from build123d import *

# Parameters (mm, degrees)
SKETCH2_R           = 100
SKETCH2_R_2         = 4
BOSS_EXTRUDE1_DEPTH = 2
SKETCH3_R           = 65
SKETCH3_R_2         = 61
CUT_EXTRUDE2_DEPTH  = 1
CUT_EXTRUDE3_DEPTH  = 10


with BuildPart() as part:
    # Sketch2 → Boss-Extrude1 (new, symmetric)
    with BuildSketch(Plane(origin=(0, 0, 0), x_dir=(1, 0, 0), z_dir=(0, 1, 0))):
        with Locations(Location((0, 0, 0), (0, 0, 270))):
            Circle(SKETCH2_R)
        with Locations(Location((50, 0, 0), (0, 0, 270))):
            Circle(SKETCH2_R_2, mode=Mode.SUBTRACT)
        with Locations(Location((-25, -43.301270189, 0), (0, 0, 270))):
            Circle(SKETCH2_R_2, mode=Mode.SUBTRACT)
        with Locations(Location((-25, 43.301270189, 0), (0, 0, 270))):
            Circle(SKETCH2_R_2, mode=Mode.SUBTRACT)
        with BuildLine():
            ThreePointArc((-36.718407842, 33.937568056), (-17.5, 30.310889132), (-11.031592158, 48.767858006))
            ThreePointArc((-11.031592158, 48.767858006), (25, 43.301270189), (47.75, 14.83028995))
            ThreePointArc((47.75, 14.83028995), (35, 0), (47.75, -14.83028995))
            ThreePointArc((47.75, -14.83028995), (25, -43.301270189), (-11.031592158, -48.767858006))
            ThreePointArc((-11.031592158, -48.767858006), (-17.5, -30.310889132), (-36.718407842, -33.937568056))
            ThreePointArc((-36.718407842, -33.937568056), (-50, 0), (-36.718407842, 33.937568056))
        make_face(mode=Mode.SUBTRACT)
    extrude(amount=BOSS_EXTRUDE1_DEPTH, both=True)

    # Sketch3 → Cut-Extrude2 (cut)
    with BuildSketch(Plane(origin=(0, 2, 0), x_dir=(1, 0, 0), z_dir=(0, 1, 0))):
        with Locations(Location((0, 0, 0), (0, 0, 270))):
            Circle(SKETCH3_R)
        with Locations(Location((0, 0, 0), (0, 0, 270))):
            Circle(SKETCH3_R_2, mode=Mode.SUBTRACT)
    extrude(amount=-CUT_EXTRUDE2_DEPTH, mode=Mode.SUBTRACT)

    # Sketch4 → Cut-Extrude3 (cut)
    with BuildSketch(Plane(origin=(0, 2, 0), x_dir=(1, 0, 0), z_dir=(0, 1, 0))):
        with BuildLine():
            Line((6.221861376, 81.776580022), (7.721861376, 84.374656233))
            ThreePointArc((7.721861376, 84.374656233), (11.819937588, 85.472732444), (12.918013799, 81.374656233))
            Line((12.918013799, 81.374656233), (11.418013799, 78.776580022))
            ThreePointArc((11.418013799, 78.776580022), (7.319937588, 77.67850381), (6.221861376, 81.776580022))
        make_face()
        with BuildLine():
            Line((0.221861376, 71.384275176), (1.721861376, 73.982351387))
            ThreePointArc((1.721861376, 73.982351387), (5.819937588, 75.080427599), (6.918013799, 70.982351387))
            Line((6.918013799, 70.982351387), (5.418013799, 68.384275176))
            ThreePointArc((5.418013799, 68.384275176), (1.319937588, 67.286198965), (0.221861376, 71.384275176))
        make_face()
        with BuildLine():
            Line((18.918013799, 91.766961078), (17.418013799, 89.168884867))
            ThreePointArc((17.418013799, 89.168884867), (13.319937588, 88.070808656), (12.221861376, 92.168884867))
            Line((12.221861376, 92.168884867), (13.721861376, 94.766961078))
            ThreePointArc((13.721861376, 94.766961078), (17.819937588, 95.86503729), (18.918013799, 91.766961078))
        make_face()
        with BuildLine():
            Line((-53.425253905, 62.224294646), (-54.20171104, 65.122072125))
            ThreePointArc((-54.20171104, 65.122072125), (-52.080390696, 68.796306739), (-48.406156082, 66.674986396))
            Line((-48.406156082, 66.674986396), (-47.629698947, 63.777208917))
            ThreePointArc((-47.629698947, 63.777208917), (-49.75101929, 60.102974303), (-53.425253905, 62.224294646))
        make_face()
        with BuildLine():
            Line((-50.319425363, 50.633184731), (-51.095882499, 53.53096221))
            ThreePointArc((-51.095882499, 53.53096221), (-48.974562155, 57.205196824), (-45.300327541, 55.08387648))
            Line((-45.300327541, 55.08387648), (-44.523870406, 52.186099001))
            ThreePointArc((-44.523870406, 52.186099001), (-46.645190749, 48.511864387), (-50.319425363, 50.633184731))
        make_face()
        with BuildLine():
            Line((-51.511984623, 78.266096311), (-50.735527488, 75.368318832))
            ThreePointArc((-50.735527488, 75.368318832), (-52.856847832, 71.694084218), (-56.531082446, 73.815404562))
            Line((-56.531082446, 73.815404562), (-57.307539581, 76.713182041))
            ThreePointArc((-57.307539581, 76.713182041), (-55.186219238, 80.387416655), (-51.511984623, 78.266096311))
        make_face()
        with BuildLine():
            Line((-81.776580022, 6.221861376), (-84.374656233, 7.721861376))
            ThreePointArc((-84.374656233, 7.721861376), (-85.472732444, 11.819937588), (-81.374656233, 12.918013799))
            Line((-81.374656233, 12.918013799), (-78.776580022, 11.418013799))
            ThreePointArc((-78.776580022, 11.418013799), (-77.67850381, 7.319937588), (-81.776580022, 6.221861376))
        make_face()
        with BuildLine():
            Line((-71.384275176, 0.221861376), (-73.982351387, 1.721861376))
            ThreePointArc((-73.982351387, 1.721861376), (-75.080427599, 5.819937588), (-70.982351387, 6.918013799))
            Line((-70.982351387, 6.918013799), (-68.384275176, 5.418013799))
            ThreePointArc((-68.384275176, 5.418013799), (-67.286198965, 1.319937588), (-71.384275176, 0.221861376))
        make_face()
        with BuildLine():
            Line((-91.766961078, 18.918013799), (-89.168884867, 17.418013799))
            ThreePointArc((-89.168884867, 17.418013799), (-88.070808656, 13.319937588), (-92.168884867, 12.221861376))
            Line((-92.168884867, 12.221861376), (-94.766961078, 13.721861376))
            ThreePointArc((-94.766961078, 13.721861376), (-95.86503729, 17.819937588), (-91.766961078, 18.918013799))
        make_face()
        with BuildLine():
            Line((-62.224294646, -53.425253905), (-65.122072125, -54.20171104))
            ThreePointArc((-65.122072125, -54.20171104), (-68.796306739, -52.080390696), (-66.674986396, -48.406156082))
            Line((-66.674986396, -48.406156082), (-63.777208917, -47.629698947))
            ThreePointArc((-63.777208917, -47.629698947), (-60.102974303, -49.75101929), (-62.224294646, -53.425253905))
        make_face()
        with BuildLine():
            Line((-50.633184731, -50.319425363), (-53.53096221, -51.095882499))
            ThreePointArc((-53.53096221, -51.095882499), (-57.205196824, -48.974562155), (-55.08387648, -45.300327541))
            Line((-55.08387648, -45.300327541), (-52.186099001, -44.523870406))
            ThreePointArc((-52.186099001, -44.523870406), (-48.511864387, -46.645190749), (-50.633184731, -50.319425363))
        make_face()
        with BuildLine():
            Line((-78.266096311, -51.511984623), (-75.368318832, -50.735527488))
            ThreePointArc((-75.368318832, -50.735527488), (-71.694084218, -52.856847832), (-73.815404562, -56.531082446))
            Line((-73.815404562, -56.531082446), (-76.713182041, -57.307539581))
            ThreePointArc((-76.713182041, -57.307539581), (-80.387416655, -55.186219238), (-78.266096311, -51.511984623))
        make_face()
        with BuildLine():
            Line((-6.221861376, -81.776580022), (-7.721861376, -84.374656233))
            ThreePointArc((-7.721861376, -84.374656233), (-11.819937588, -85.472732444), (-12.918013799, -81.374656233))
            Line((-12.918013799, -81.374656233), (-11.418013799, -78.776580022))
            ThreePointArc((-11.418013799, -78.776580022), (-7.319937588, -77.67850381), (-6.221861376, -81.776580022))
        make_face()
        with BuildLine():
            Line((-0.221861376, -71.384275176), (-1.721861376, -73.982351387))
            ThreePointArc((-1.721861376, -73.982351387), (-5.819937588, -75.080427599), (-6.918013799, -70.982351387))
            Line((-6.918013799, -70.982351387), (-5.418013799, -68.384275176))
            ThreePointArc((-5.418013799, -68.384275176), (-1.319937588, -67.286198965), (-0.221861376, -71.384275176))
        make_face()
        with BuildLine():
            Line((-18.918013799, -91.766961078), (-17.418013799, -89.168884867))
            ThreePointArc((-17.418013799, -89.168884867), (-13.319937588, -88.070808656), (-12.221861376, -92.168884867))
            Line((-12.221861376, -92.168884867), (-13.721861376, -94.766961078))
            ThreePointArc((-13.721861376, -94.766961078), (-17.819937588, -95.86503729), (-18.918013799, -91.766961078))
        make_face()
        with BuildLine():
            Line((53.425253905, -62.224294646), (54.20171104, -65.122072125))
            ThreePointArc((54.20171104, -65.122072125), (52.080390696, -68.796306739), (48.406156082, -66.674986396))
            Line((48.406156082, -66.674986396), (47.629698947, -63.777208917))
            ThreePointArc((47.629698947, -63.777208917), (49.75101929, -60.102974303), (53.425253905, -62.224294646))
        make_face()
        with BuildLine():
            Line((50.319425363, -50.633184731), (51.095882499, -53.53096221))
            ThreePointArc((51.095882499, -53.53096221), (48.974562155, -57.205196824), (45.300327541, -55.08387648))
            Line((45.300327541, -55.08387648), (44.523870406, -52.186099001))
            ThreePointArc((44.523870406, -52.186099001), (46.645190749, -48.511864387), (50.319425363, -50.633184731))
        make_face()
        with BuildLine():
            Line((51.511984623, -78.266096311), (50.735527488, -75.368318832))
            ThreePointArc((50.735527488, -75.368318832), (52.856847832, -71.694084218), (56.531082446, -73.815404562))
            Line((56.531082446, -73.815404562), (57.307539581, -76.713182041))
            ThreePointArc((57.307539581, -76.713182041), (55.186219238, -80.387416655), (51.511984623, -78.266096311))
        make_face()
        with BuildLine():
            Line((81.776580022, -6.221861376), (84.374656233, -7.721861376))
            ThreePointArc((84.374656233, -7.721861376), (85.472732444, -11.819937588), (81.374656233, -12.918013799))
            Line((81.374656233, -12.918013799), (78.776580022, -11.418013799))
            ThreePointArc((78.776580022, -11.418013799), (77.67850381, -7.319937588), (81.776580022, -6.221861376))
        make_face()
        with BuildLine():
            Line((71.384275176, -0.221861376), (73.982351387, -1.721861376))
            ThreePointArc((73.982351387, -1.721861376), (75.080427599, -5.819937588), (70.982351387, -6.918013799))
            Line((70.982351387, -6.918013799), (68.384275176, -5.418013799))
            ThreePointArc((68.384275176, -5.418013799), (67.286198965, -1.319937588), (71.384275176, -0.221861376))
        make_face()
        with BuildLine():
            Line((91.766961078, -18.918013799), (89.168884867, -17.418013799))
            ThreePointArc((89.168884867, -17.418013799), (88.070808656, -13.319937588), (92.168884867, -12.221861376))
            Line((92.168884867, -12.221861376), (94.766961078, -13.721861376))
            ThreePointArc((94.766961078, -13.721861376), (95.86503729, -17.819937588), (91.766961078, -18.918013799))
        make_face()
        with BuildLine():
            Line((62.224294646, 53.425253905), (65.122072125, 54.20171104))
            ThreePointArc((65.122072125, 54.20171104), (68.796306739, 52.080390696), (66.674986396, 48.406156082))
            Line((66.674986396, 48.406156082), (63.777208917, 47.629698947))
            ThreePointArc((63.777208917, 47.629698947), (60.102974303, 49.75101929), (62.224294646, 53.425253905))
        make_face()
        with BuildLine():
            Line((50.633184731, 50.319425363), (53.53096221, 51.095882499))
            ThreePointArc((53.53096221, 51.095882499), (57.205196824, 48.974562155), (55.08387648, 45.300327541))
            Line((55.08387648, 45.300327541), (52.186099001, 44.523870406))
            ThreePointArc((52.186099001, 44.523870406), (48.511864387, 46.645190749), (50.633184731, 50.319425363))
        make_face()
        with BuildLine():
            Line((78.266096311, 51.511984623), (75.368318832, 50.735527488))
            ThreePointArc((75.368318832, 50.735527488), (71.694084218, 52.856847832), (73.815404562, 56.531082446))
            Line((73.815404562, 56.531082446), (76.713182041, 57.307539581))
            ThreePointArc((76.713182041, 57.307539581), (80.387416655, 55.186219238), (78.266096311, 51.511984623))
        make_face()
    extrude(amount=-CUT_EXTRUDE3_DEPTH, mode=Mode.SUBTRACT)


solid = part.part
Model file for the job. Use its own axes, mm. A direction names the side the tool comes from. Round coordinates to 2 decimals unless told otherwise and drop trailing zeros. Loops run counter-clockwise (first coordinate to the right, second up) from the corner with the lowest first, then second, coordinate; pieces in that order, holes last. Notation, with made-up numbers: M 87.5,47.5 L 143.5,47.5 A26 cw 143.5,86.5 Z; hole C 16,35.5 d5. An arc over 180 degrees is marked long. One line per question, with ' | ' between items.
1) Drill centre lines: line 1 along X through (y, z) = (1.5, 27); line 2 along X through (y, z) = (1.6, -9); line 3 along Z through (x, y) = (-56, -0.95). Where is each one in solid material? Low to high.
Solved:
line 1: x = -96.29 to -59.13, -54.7 to -42.08, 42.08 to 54.7, 59.13 to 96.29 | line 2: x = -99.59 to -85.57, -77.28 to -64.37, -60.33 to -49.18, 38 to 60.33, 64.37 to 99.59 | line 3: z = -82.85 to -80.03, -72.75 to 45.72, 50.68 to 82.85
2) Band-saw the part on A-A (x = 28). Give the cut face in (y, z), then the cut area to 3 significant figures.
Solved:
outline: M -2,-96 L 2,-96 L 2,-58.66 L 1,-58.66 L 1,-54.19 L 2,-54.19 L 2,-41.42 L -2,-41.42 Z; M -2,41.42 L 2,41.42 L 2,54.19 L 1,54.19 L 1,58.66 L 2,58.66 L 2,96 L -2,96 Z | area: 428 mm²
3) Band-saw the part on C-C (x = -33). Give the cut face in (y, z), then the cut area to 3 significant figures.
Solved:
outline: M -2,-94.4 L 2,-94.4 L 2,-56 L 1,-56 L 1,-51.3 L 2,-51.3 L 2,-30.61 L -2,-30.61 Z; M -2,30.61 L 2,30.61 L 2,51.3 L 1,51.3 L 1,56 L 2,56 L 2,94.4 L -2,94.4 Z | area: 501 mm²
4) Flat gauge pin, fed straight in: pin 1 (2 mm diameter, centred on y = 0, z = -55, fed in from +X). Where does the tip first touch, or does it go through?
Solved:
pin 1: stops at x = 84.17
5) 3-axis set-ups, long thin cutter, end or side, ignore diameter. For faces 1 (the cylindrical face through (-85.505, 0.028, -11.762)), 2 (the flat face through (58, 1, -20)): which of +Z, -Z, +X, -X, +Y, -Y reach the whole face in a straight line?
Solved:
face 1: +Y, -Y | face 2: +Y
6) Band-saw the part on B-B (y = 0.05). Give the number of separate pieces and of enclosed holes in the cut face, then the cut area to 3 significant figures.
Solved:
separate pieces: 1 | enclosed holes: 28 | area: 23,300 mm²
7) Mould opens along Z. For faces 3 (the cylindrical face through (13.377, 0.028, -88.038)), 4 (the cylindrical face through (19.52, 1.51, 62)), 5 (the flat face through (-20.8, -2, 43)) say: +Z half, -Z half, draft (parallel to the pull), parting line (faces both ways), or undercut.
Solved:
face 3: undercut | face 4: undercut | face 5: draft
